Can you work these out from the drawing? Everything is in mm from the part's minimum corner. Coordinates: 2 decimals unless noted, no trailing zeros. Return JSON: item names as keys, results as strings. Group by question number.
1) Thinking about a two-plate mould opening in X: for the marked faces 1, 2, 3 and 4, which applies, +X half, -X half, draft (parallel to the pull), parting line (faces both ways), or undercut?
2) If I drill on probe 1 along X at (y, z) = (9.5, 18) (1 decimal); probe 2 along X at (y, z) = (5.5, 13); probe 3 along X at (y, z) = (4.75, 15.5), over which ranges is the centre line in solid material (lowest first)? Write a range as from..to.
3) For pin 1 (0.5 mm diameter, centred on x = 61, y = 14.5, fed in from +Z); pin 2 (8 mm diameter, centred on x = 82.55, y = 4.445, fed in from +Z), each with a flat end and sliding along its axis, tell me the tip position at first contact or that it passes through.
4) If we section it at B-B, the plane z = 8: State how many separate pieces and enclosed holes the cut face has, then the cut area to 3 significant figures.
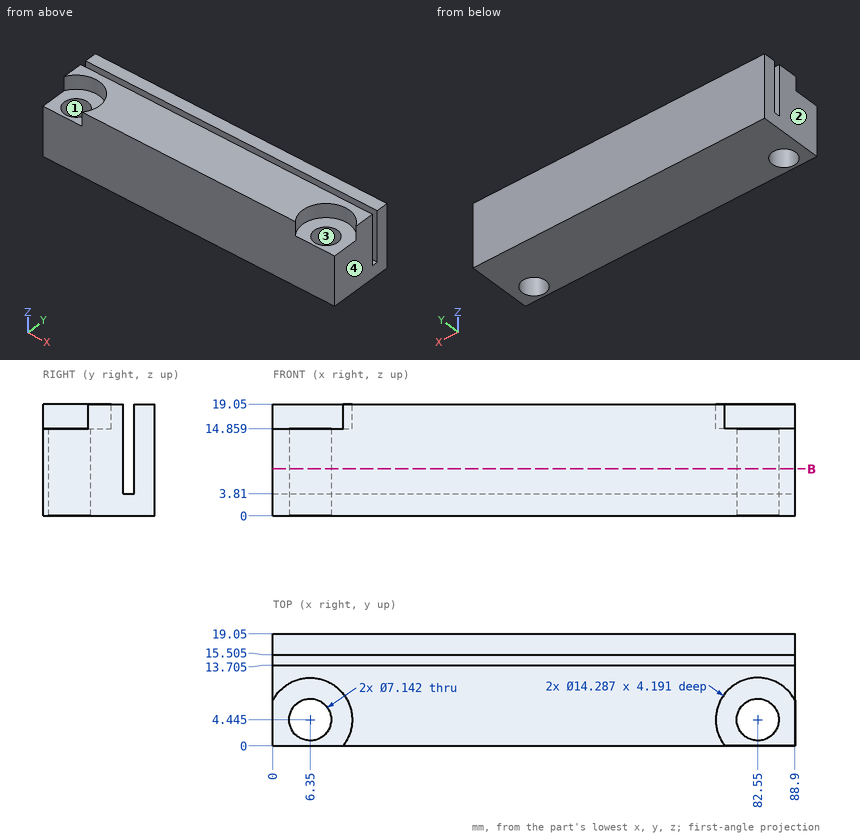
Result sheet:
{
 "1": {"face 1": "undercut", "face 2": "-X half", "face 3": "undercut", "face 4": "+X half"},
 "2": {"probe 1": "x = 0..1.3, 11.4..77.5, 87.6..88.9", "probe 2": "x = 0..2.94, 9.76..79.14, 85.96..88.9", "probe 3": "x = 13.49..75.41"},
 "3": {"pin 1": "stops at z = 3.81", "pin 2": "stops at z = 14.86"},
 "4": {"separate pieces": "2", "enclosed holes": "2", "area": "1,450 mm2"}
}
